Source: CAD feature listing. Evaluate the final solid. Frame: model axes, mm. A direction names the side the tool comes from. Round coordinates to 2 decimals unless told otherwise and drop trailing zeros. Loops run counter-clockwise (first coordinate to the right, second up) from the corner with the lowest first, then second, coordinate; pieces in that order, holes last. Notation, with made-up numbers: M 84,51.25 L 130,51.25 A22 ccw 130,66.25 Z; hole C 7,-15.5 d5. An arc over 180 degrees is marked long. Answer as CSV lines item,"result". Start each with the question number.
```python
from build123d import *

# Parameters (mm, degrees)
DODANIE_WYCI_GNI_CIE1_DEPTH = 125
DODANIE_WYCI_GNI_CIE3_DEPTH = 10
SZKIC4_R                    = 10
WYTNIJ_WYCI_GNI_CIE1_DEPTH  = 10


with BuildPart() as part:
    # Szkic2 → Dodanie-wyciągnięcie1 (new body)
    with BuildSketch(Plane.XY):
        Polygon((0, 0), (0, 65), (10, 65), (10, 10), (75, 10), (75, 0), align=None)
    extrude(amount=-DODANIE_WYCI_GNI_CIE1_DEPTH)

    # Szkic3 → Dodanie-wyciągnięcie3 (add)
    with BuildSketch(Plane.XY):
        Polygon((10, 65), (75, 10), (10, 10), align=None)
    extrude(amount=-DODANIE_WYCI_GNI_CIE3_DEPTH)

    # Szkic4 → Wytnij-wyciągnięcie1 (cut)
    with BuildSketch(Plane(origin=(0, 10, 0), x_dir=(1, 0, 0), z_dir=(0, 1, 0))):
        with Locations(Location((50, 62.5, 0), (0, 0, 180))):
            Circle(SZKIC4_R)
    extrude(amount=-WYTNIJ_WYCI_GNI_CIE1_DEPTH, mode=Mode.SUBTRACT)


solid = part.part
```
1) Access query for faces 1 (the flat face through (38, 0, -62)), 2 (the flat face through (29, 26, -10)). Directions: +Z, -Z, +X, -X, +Y, -Y. A direction counts if a zero-diameter tool reaches every point of the face in a straight line with its end or side. Return the directions, or none.
2) Contact query for flat-ended pins moving along their axis: pin 1 Ø4 at (x, z) = (33, -89.5) entering from +Y; pin 2 Ø12 at (x, z) = (50, -62.5) entering from -Y; pin 3 Ø3 at (y, z) = (31.5, -43.5) entering from +X. Output: stop coordinate, or through.
3) Section A-A, the plane z = -56.5. Return loops of the section in (x, y), and give its area (3 significant figures).
4) Section D-D, the plane y = 35. Return loops of the section in (x, z), and give its area (3 significant figures).
5) Ray query, line 1 along Z through (x, y) = (50, 6.75); line 2 along X through (y, z) = (3, -62); line 3 along Y through (x, z) = (40, -77). Return the intervals inside material, ascending.
6) Mould query, pull axis X, two halves, no side actions, for faces 3 (the cylindrical face through (57.94, 5.07, -68.58)), 4 (the flat face through (0, 32, -62)), 5 (the flat face through (75, 5, -62)), 6 (the flat face through (5, 65, -62)). Classes: pulls with the +X half, pulls with the -X half, needs draft (parallel to the pull), parting line crosses it, or undercut.
7) Section B-B, the plane x = 50. Return loops of the section in (y, z), and give its area (3 significant figures).
8) Section C-C, the plane z = -108. Return loops of the section in (x, y), and give its area (3 significant figures).
Findings below:
1,face 1,"+Z, -Z, +X, -X, -Y"
1,face 2,"-Z, +X, +Y"
2,pin 1,"y = 10"
2,pin 2,"through"
2,pin 3,"x = 10"
3,outline,"M 0,0 L 42,0 L 42,10 L 10,10 L 10,65 L 0,65 Z; M 58,0 L 75,0 L 75,10 L 58,10 Z"
3,area,"1,140 mm²"
4,outline,"M 0,-125 L 10,-125 L 10,-10 L 45.45,-10 L 45.45,0 L 0,0 Z"
4,area,"1,600 mm²"
5,line 1,"-125 to -72.5, -52.5 to 0"
5,line 2,"0 to 40.01, 59.99 to 75"
5,line 3,"0 to 10"
6,face 3,"undercut"
6,face 4,"pulls with the -X half"
6,face 5,"pulls with the +X half"
6,face 6,"needs draft"
7,outline,"M 0,-125 L 10,-125 L 10,-72.5 L 0,-72.5 Z; M 0,-52.5 L 10,-52.5 L 10,-10 L 31.15,-10 L 31.15,0 L 0,0 Z"
7,area,"1,260 mm²"
8,outline,"M 0,0 L 75,0 L 75,10 L 10,10 L 10,65 L 0,65 Z"
8,area,"1,300 mm²"
